The listing builds one solid part. Answer for the finished solid, in the listing's coordinates (mm). Face numbers are marked on the shaded views. A direction names the side the tool comes from. Give positions to 0.01 mm unless a question says otherwise; leave off trailing zeros. Write each loop counter-clockwise with the first axis right and the second up, starting at its lowest first coordinate (ties: lowest second). Pieces come first, ordered by that corner, then holes. Notation, with made-up numbers: M 41.25,-19 L 85.25,-19 A11 cw 85.25,-12 Z; hole C 60.25,25.5 d8. An arc over 180 degrees is marked long. Answer as a JSON object with one key per item and string values.
```python
from build123d import *

# Parameters (mm, degrees)
ESQUISSE1_R             = 5
BOSS_EXTRU_1_DEPTH      = 3.2
BOSS_EXTRU_2_START      = 3.2
ESQUISSE1_3_R           = 4.4
BOSS_EXTRU_2_DEPTH      = 0.8
BOSS_EXTRU_3_DEPTH      = 8.1
ENL_V_START             = 4
ESQUISSE1_5_R           = 2.75
ENL_V_MAT_EXTRU_1_DEPTH = 9
BOSS_EXTRU_4_START      = -5
ESQUISSE1_6_R           = 0.95
BOSS_EXTRU_4_DEPTH      = 6.9
CHANFREIN1_SIZE         = 1
CONG_1_R                = 0.95
ESQUISSE2_W             = 0.6
ESQUISSE2_H             = 2.3
BOSS_EXTRU_5_DEPTH      = 6.1
ESQUISSE2_3_W           = 0.6
ESQUISSE2_3_H           = 2.3
BOSS_EXTRU_6_DEPTH      = 4.7
CONG_2_R                = 1.15
ENL_V_MAT_EXTRU_2_REACH = 18.731
ESQUISSE3_R             = 0.6
ENL_V_MAT_EXTRU_3_REACH = 19.001
ESQUISSE4_R             = 0.6


with BuildPart() as part:
    # Esquisse1 → Boss.-Extru.1 (new body)
    with BuildSketch(Plane.XY):
        Circle(ESQUISSE1_R)
    extrude(amount=BOSS_EXTRU_1_DEPTH)

    # Esquisse1<3> → Boss.-Extru.2 (add)
    with BuildSketch(Plane.XY.offset(BOSS_EXTRU_2_START)):
        Circle(ESQUISSE1_3_R)
    extrude(amount=BOSS_EXTRU_2_DEPTH)

    # Esquisse1<4> → Boss.-Extru.3 (add)
    with BuildSketch(Plane.XY):
        with BuildLine():
            Line((-1.559647396, 3.3), (1.559647396, 3.3))
            ThreePointArc((1.559647396, 3.3), (3.65, 0), (1.559647396, -3.3))
            Line((1.559647396, -3.3), (-1.559647396, -3.3))
            ThreePointArc((-1.559647396, -3.3), (-3.65, 0), (-1.559647396, 3.3))
        make_face()
    extrude(amount=-BOSS_EXTRU_3_DEPTH)

    # Esquisse1<5> → Enlèv. mat.-Extru.1 (cut)
    with BuildSketch(Plane.XY.offset(ENL_V_START)):
        Circle(ESQUISSE1_5_R)
    extrude(amount=-ENL_V_MAT_EXTRU_1_DEPTH, mode=Mode.SUBTRACT)

    # Esquisse1<6> → Boss.-Extru.4 (add)
    with BuildSketch(Plane.XY.offset(BOSS_EXTRU_4_START)):
        Circle(ESQUISSE1_6_R)
    extrude(amount=BOSS_EXTRU_4_DEPTH)

    # Chanfrein1
    chanfrein1_edges = [part.edges().sort_by_distance(p)[0] for p in [
        (-2.75, 0, 4),
    ]]
    chamfer(chanfrein1_edges, length=CHANFREIN1_SIZE)

    # Congé1
    cong_1_edges = [part.edges().sort_by_distance(p)[0] for p in [
        (-0.95, 0, 1.9),
    ]]
    fillet(cong_1_edges, radius=CONG_1_R)

    # Esquisse2 → Boss.-Extru.5 (add)
    with BuildSketch(Plane(origin=(0, 0, -8.1), x_dir=(-1, 0, 0), z_dir=(0, 0, -1))):
        with Locations((-2.6, 0)):
            Rectangle(ESQUISSE2_W, ESQUISSE2_H)
    extrude(amount=BOSS_EXTRU_5_DEPTH)

    # Esquisse2<3> → Boss.-Extru.6 (add)
    with BuildSketch(Plane(origin=(0, 0, -8.1), x_dir=(-1, 0, 0), z_dir=(0, 0, -1))):
        with Locations((2.6, 0)):
            Rectangle(ESQUISSE2_3_W, ESQUISSE2_3_H)
    extrude(amount=BOSS_EXTRU_6_DEPTH)

    # Congé2
    cong_2_edges = [part.edges().sort_by_distance(p)[0] for p in [
        (-2.6, -1.15, -12.8),
        (-2.6, 1.15, -12.8),
        (2.6, -1.15, -14.2),
        (2.6, 1.15, -14.2),
    ]]
    fillet(cong_2_edges, radius=CONG_2_R - 0.0001)  # a hair under: the kernel refuses the full size

    # Esquisse3 → Enlèv. mat.-Extru.2 (cut, up to next)
    with BuildSketch(Plane.ZY.offset(-2.3), mode=Mode.PRIVATE) as enl_v_mat_extru_2_sk1:
        with Locations((-13.05, 0)):
            Circle(ESQUISSE3_R)
    enl_v_mat_extru_2_tool1 = extrude(enl_v_mat_extru_2_sk1.sketch, amount=-ENL_V_MAT_EXTRU_2_REACH, mode=Mode.PRIVATE) & part.part
    add(enl_v_mat_extru_2_tool1.solids().sort_by_distance((2.3, 0, -13.05))[0], mode=Mode.SUBTRACT)

    # Esquisse4 → Enlèv. mat.-Extru.3 (cut, up to next)
    with BuildSketch(Plane.ZY.offset(2.9), mode=Mode.PRIVATE) as enl_v_mat_extru_3_sk1:
        with Locations(Location((-11.65, 0, 0), (0, 0, 270))):
            Circle(ESQUISSE4_R)
    enl_v_mat_extru_3_tool1 = extrude(enl_v_mat_extru_3_sk1.sketch, amount=-ENL_V_MAT_EXTRU_3_REACH, mode=Mode.PRIVATE) & part.part
    add(enl_v_mat_extru_3_tool1.solids().sort_by_distance((-2.9, 0, -11.65))[0], mode=Mode.SUBTRACT)


solid = part.part
```
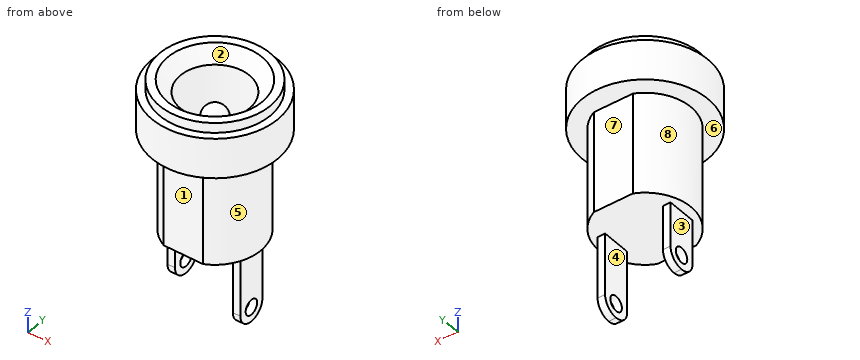
1. For the marked faces 4, 5, 6, 7 and 8, determine the directions among +Z, -Z, +X, -X, +Y, -Y from which every point of the face is accessible in a straight line to the end or side of a thin tool.
Verdict:
{"face 4": "-Z, +Y, -Y", "face 5": "-Z, +X", "face 6": "-Z", "face 7": "-Z, +X, -X, +Y", "face 8": "-Z, -X"}
2. The mould has two halves that part along X. Classify the marked faces 1, 2 and 3: released by +X, released by -X, zero draft, split by the parting line, or undercut.
Verdict:
{"face 1": "zero draft", "face 2": "undercut", "face 3": "released by -X"}
3. A cutting plane is placed at C-C, the plane x = 4. Give the vertices of the cut face in (y, z), plus the area to 3 significant figures.
Verdict:
{"outline": "M -3,0 L 3,0 L 3,3.2 L 1.83,3.2 L 1.83,4 L -1.83,4 L -1.83,3.2 L -3,3.2 Z", "area": "22.1 mm2"}
4. A cutting plane is placed at D-D, the plane z = 1.5. Give the vertices of the cut face in (x, y).
Verdict:
{"outline": "C 0,0 d10; C 0,0 d1.55; hole C 0,0 d5.5"}
5. A cutting plane is placed at A-A, the plane z = -4.5. Give the vertices of the cut face in (x, y), plus the area to 3 significant figures.
Verdict:
{"outline": "M -1.56,-3.3 L 1.56,-3.3 A3.65 ccw 1.56,3.3 L -1.56,3.3 A3.65 ccw Z; C 0,0 d1.9; hole C 0,0 d5.5", "area": "19.5 mm2"}
6. Flat-ended cylindrical pins translate along their axes: pin 1 (3 mm diameter, centred on x = -1, y = 0.5, fed in from +Z); pin 2 (1.1 mm diameter, centred on y = 0, z = -11.65, fed in from +X); pin 3 (2 mm diameter, centred on x = -1.5, y = 1.5, fed in from +Z). Find the tip coordinate at first contact, or state that the pin passes through.
Verdict:
{"pin 1": "stops at z = 1.9", "pin 2": "stops at x = 2.9", "pin 3": "stops at z = 3.37"}
7. A cutting plane is placed at B-B, the plane x = 0. Give the vertices of the cut face in (y, z).
Verdict:
{"outline": "M -5,0 L -3.3,0 L -3.3,-8.1 L 3.3,-8.1 L 3.3,0 L 5,0 L 5,3.2 L 4.4,3.2 L 4.4,4 L 3.75,4 L 2.75,3 L 2.75,-5 L 0.95,-5 L 0.95,0.95 A0.95 ccw -0.95,0.95 L -0.95,-5 L -2.75,-5 L -2.75,3 L -3.75,4 L -4.4,4 L -4.4,3.2 L -5,3.2 Z"}
8. Consider line 1 along Y through (x, z) = (0, -4.5); line 2 along Y through (x, z) = (2.75, -13.05); line 3 along Y through (x, z) = (2.5, -10.5). Determine where each line is inside the solid, lowest interval first.
Verdict:
{"line 1": "y = -3.3 to -2.75, -0.95 to 0.95, 2.75 to 3.3", "line 2": "y = -1.15 to -0.6, 0.6 to 1.15", "line 3": "y = -1.15 to 1.15"}
